Can you work these out from the model? Positions are in its coordinate system, mm. A direction names the side the tool comes from. Round coordinates to 2 decimals unless told otherwise and drop trailing zeros. Write each loop counter-clockwise with the first axis right and the second up, starting at its lowest first coordinate (ties: lowest second). Pieces come first, ordered by that corner, then holes. Notation, with made-up numbers: (-35.75, 47) - (18.25, 47) arc R28 cw to (18.25, 73) - close; hole circle Ø7 at (47.25, 4.25). An arc over 180 degrees is marked (long way). One line per item, written item: value. Start each with the question number.
(1) I want a section at D-D on x = 4. List the corners of the cut face in (y, z) for me, plus the area to 3 significant figures.
(2) If I drill on L1, parallel to X at y = 55.5, z = 26; L2, parallel to Z at x = 32.35, y = 57; L3, parallel to Y at x = 2.5, z = 26, over which ranges is the centre line in solid material (lowest first)? Write a range as from..to.
(3) Thinking about a two-plate mould opening in Z: for faces 3 (the face through (58.35, 55, 26)), 4 (the face through (5, 42, 0)), 5 (the face through (17.57, 55.13, 32.13)), 6 (the face through (5, 42, 52)), which applies, +Z half, -Z half, draft (parallel to the pull), parting line (faces both ways), or undercut?
(4) I want a section at C-C on z = 22.5. List the corners of the cut face in (x, y) for me.
(5) I'm going to push flat-ended pins straight in: pin 1 Ø5 at (x, z) = (50, 15.5) entering from -Y; pin 2 Ø12 at (y, z) = (14, 37) entering from +X. Where does each tip first touch, or does it pass through?
(6) I want a section at B-B on y = 26. List the corners of the cut face in (x, z) for me, plus the area to 3 significant figures.
(7) I want a section at A-A on x = 32.35. List the corners of the cut face in (y, z) for me, plus the area to 3 significant figures.
(8) On a 3-axis mill with a long thin cutter (end or side, diameter ignored), from which of +Z, -Z, +X, -X, +Y, -Y can I reach the whole of each face in a straight line? I mean faces 1 (the face through (20, 52, 14)), 2 (the face through (3.22, 10.38, 29.47)). Say none if no direction works.
from build123d import *

# Parameters (mm, degrees)
BOSS_EXTRUDE1_DEPTH = 52
SKETCH2_R           = 16
CUT_EXTRUDE1_DEPTH  = 52
SKETCH3_R           = 16
CUT_EXTRUDE2_DEPTH  = 52


with BuildPart() as part:
    # Sketch1 → Boss-Extrude1 (new body)
    with BuildSketch(Plane.XY):
        Polygon((0, 0), (6.35, 0), (6.35, 52), (58.35, 52), (58.35, 58.35), (0, 58.35), (0, 32.973080538), align=None)
    extrude(amount=BOSS_EXTRUDE1_DEPTH)

    # Sketch2 → Cut-Extrude1 (cut)
    with BuildSketch(Plane(origin=(0, 52, 0), x_dir=(-1, 0, 0), z_dir=(0, -1, 0))):
        with Locations((-32.35, -26)):
            Circle(SKETCH2_R)
    extrude(amount=-CUT_EXTRUDE1_DEPTH, mode=Mode.SUBTRACT)

    # Sketch3 → Cut-Extrude2 (cut)
    with BuildSketch(Plane(origin=(6.35, 0, 0), x_dir=(0, 0, -1), z_dir=(1, 0, 0))):
        with Locations((-26, 26)):
            Circle(SKETCH3_R)
    extrude(amount=-CUT_EXTRUDE2_DEPTH, mode=Mode.SUBTRACT)


solid = part.part
Established:
1. outline: (0, 0) - (58.35, 0) - (58.35, 52) - (0, 52) - close; hole circle Ø32 at (26, 26)
1. area: 2,230 mm2
2. L1: 0..16.35, 48.35..58.35
2. L2: 0..10, 42..52
2. L3: 0..10, 42..58.35
3. face 3: draft
3. face 4: -Z half
3. face 5: undercut
3. face 6: +Z half
4. outline: (0, 0) - (6.35, 0) - (6.35, 10.39) - (0, 10.39) - close; (0, 41.61) - (6.35, 41.61) - (6.35, 52) - (16.74, 52) - (16.74, 58.35) - (0, 58.35) - close; (47.96, 52) - (58.35, 52) - (58.35, 58.35) - (47.96, 58.35) - close
5. pin 1: y = 52
5. pin 2: x = 6.35
6. outline: (0, 0) - (6.35, 0) - (6.35, 10) - (0, 10) - close; (0, 42) - (6.35, 42) - (6.35, 52) - (0, 52) - close
6. area: 127 mm2
7. outline: (52, 0) - (58.35, 0) - (58.35, 10) - (52, 10) - close; (52, 42) - (58.35, 42) - (58.35, 52) - (52, 52) - close
7. area: 127 mm2
8. face 1: +Z, -Z, +X, -Y
8. face 2: +X, -X
